Check sheet for the modelled part. Datum: model origin and axes. Units: mm. Face numbers are marked on the shaded views. Give positions to 0.01 mm unless a question says otherwise; leave off trailing zeros. Order: outer loops, then holes, each group sorted by start corner. A loop starts at its lowest first (then second) coordinate and runs counter-clockwise, first axis right, second up. Notation, with made-up numbers: (-27.75, -19.5) -> (26.25, -19.5) arc R25 cw to (26.25, 18.5) -> close; hole circle Ø9 at (-9, 50). An arc over 180 degrees is marked (long way). Answer in a Markdown table with one row per item. Add a question column.
(1) Go/stop test with flat-tipped pins: pin 1 (10 mm diameter, centred on y = 25, z = -4, fed in from +X); pin 2 (4 mm diameter, centred on y = 65, z = -6.5, fed in from -X); pin 3 (4 mm diameter, centred on x = 38, z = -4.5, fed in from -Y); pin 4 (1 mm diameter, centred on x = 30.5, z = -5.5, fed in from +Y). Record where each tip stops, or that it passes through.
(2) Thickness scan on L1, parallel to Y at x = 28.5, z = 2.5; L2, parallel to Y at x = -18.3, z = -4; L3, parallel to Z at x = 38.2, y = 62.3 (3 decimals). Record the ranges inside material, lowest first. Write a range as [from, to].
(3) Cross-section at A-A (x = 18.9). Record the cut outline in (y, z) (3 decimals), then the cut area to 3 significant figures.
(4) Cross-section at C-C (x = 27.5). Record the cut outline in (y, z) (3 decimals), then the cut area to 3 significant figures.
(5) Release check for a two-part mould opening along Y. For the marked faces 1, 2 and 3 record: released by +Y, released by -Y, zero draft, split by the parting line, or undercut.
(6) Cross-section at D-D (y = 23). Record the cut outline in (x, z), then the cut area to 3 significant figures.
(7) Cross-section at B-B (y = 39). Record the cut outline in (x, z).
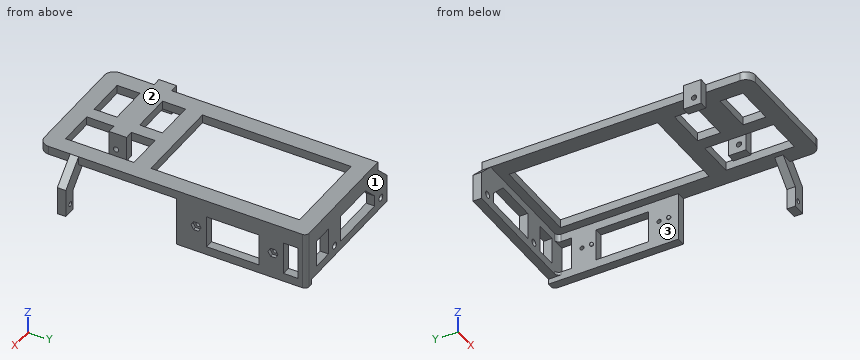
```python
from build123d import *

# Parameters (mm, degrees)
EXTRUDE_5_DEPTH      = 4
SKETCH_5_W           = 65.55
SKETCH_5_H           = 20.755
SKETCH_5_R           = 1.55
EXTRUDE_6_DEPTH      = 4
SKETCH_7_W           = 65.55
SKETCH_7_H           = 126.45
EXTRUDE_8_DEPTH      = 4
SKETCH_11_W          = 17.25
SKETCH_11_H          = 32.3
SKETCH_11_W_2        = 18.8
SKETCH_11_H_2        = 10.8
CUT_EXTRUDE_3_DEPTH  = 125.085535116
EXTRUDE_9_DEPTH      = 4
CUT_EXTRUDE_4_DEPTH  = 10
SKETCH_14_W          = 9.75
SKETCH_14_H          = 12.755
CUT_EXTRUDE_5_DEPTH  = 10
SKETCH_16_W          = 15.255
SKETCH_16_H          = 24.75
SKETCH_16_W_2        = 15.505
SKETCH_16_H_2        = 6.88
CUT_EXTRUDE_6_DEPTH  = 133.101854737
EXTRUDE_2_DEPTH      = 4
CUT_EXTRUDE_7_REACH  = 127.39
SKETCH_19_R          = 1.1
SKETCH_21_W          = 4
SKETCH_21_H          = 2.5
EXTRUDE_11_DEPTH     = 4
FILLET_2_R           = 2
FILLET_3_R           = 4.65
SKETCH_24_R          = 1
CUT_EXTRUDE_10_DEPTH = 133.101854737
SKETCH_25_R          = 0.9
EXTRUDE_12_DEPTH     = 1
FILLET_4_R           = 0.8
CUT_EXTRUDE_11_DEPTH = 1.68


with BuildPart() as part:
    # 草图4 → 凸台-拉伸5 (new body)
    with BuildSketch(Plane(origin=(37.65, 0, 0), x_dir=(0, 0, -1), z_dir=(1, 0, 0))):
        Polygon((23.255, 110.55), (19.873443934, 110.55), (11.636556066, 110.55), (0, 110.55), (0, 53.1366), (23.255, 53.1366), align=None)
    extrude(amount=EXTRUDE_5_DEPTH)

    # 草图5 → 凸台-拉伸6 (add)
    with BuildSketch(Plane(origin=(0, 110.55, 0), x_dir=(1, 0, 0), z_dir=(0, 1, 0))):
        with Locations((8.875, 10.3775)):
            Rectangle(SKETCH_5_W, SKETCH_5_H)
        with Locations(Location((-18.9, 15.755, 0), (0, 0, 180))):
            Circle(SKETCH_5_R, mode=Mode.SUBTRACT)
        with Locations(Location((18.9, 15.755, 0), (0, 0, 180))):
            Circle(SKETCH_5_R, mode=Mode.SUBTRACT)
    extrude(amount=EXTRUDE_6_DEPTH)

    # 草图7 → 凸台-拉伸8 (add)
    with BuildSketch(Plane.XY):
        with Locations((8.875, 51.325)):
            Rectangle(SKETCH_7_W, SKETCH_7_H)
    extrude(amount=EXTRUDE_8_DEPTH)

    # 草图11 → 切除-拉伸3 (cut, through all)
    with BuildSketch(Plane(origin=(0, 0, 0), x_dir=(-1, 0, 0), z_dir=(0, 0, -1))):
        with Locations((-25.025, 12.25)):
            Rectangle(SKETCH_11_W, SKETCH_11_H)
        Polygon((-33.65, 106.55), (-33.65, 36.4), (-16.4, 36.4), (8.4, 36.4), (8.4, 106.55), align=None)
        with Locations((-1, 1.5)):
            Rectangle(SKETCH_11_W_2, SKETCH_11_H_2)
        with Locations((-1, 23)):
            Rectangle(SKETCH_11_W_2, SKETCH_11_H_2)
        with BuildLine():
            ThreePointArc((16.4, -7.25), (15.038046533, -10.538046533), (11.75, -11.9))
            Line((11.75, -11.9), (23.9, -11.9))
            Line((23.9, -11.9), (23.9, 106.55))
            Line((23.9, 106.55), (16.4, 106.55))
            Line((16.4, 106.55), (16.4, -7.25))
        make_face()
    extrude(amount=-CUT_EXTRUDE_3_DEPTH, mode=Mode.SUBTRACT)

    # 草图12 → 凸台-拉伸9 (add)
    with BuildSketch(Plane(origin=(0, 2.890336251, 0), x_dir=(1, 0, 0), z_dir=(0, 1, 0))):
        Polygon((52.095757056, 19.755), (46.095757056, 19.755), (46.095757056, 9.855), (36.240757056, 0), (41.65, -4), (52.095757056, 6.445757056), align=None)
    extrude(amount=EXTRUDE_9_DEPTH)

    # 草图13 → 切除-拉伸4 (cut, symmetric)
    with BuildSketch(Plane.XZ.offset(-110.55)):
        Polygon((-23.9, -7.5), (-16.4, 0), (-16.4, 4), (-23.9, 4), align=None)
    extrude(amount=CUT_EXTRUDE_4_DEPTH, both=True, mode=Mode.SUBTRACT)

    # 草图14 → 切除-拉伸5 (cut)
    with BuildSketch(Plane.XZ.offset(-110.55)):
        with Locations((28.775, -10.3775)):
            Rectangle(SKETCH_14_W, SKETCH_14_H)
        Polygon((13.9, -16.755), (-13.9, -16.755), (-13.9, -11.642135624), (-6.257864376, -4), (13.9, -4), align=None)
    extrude(amount=-CUT_EXTRUDE_5_DEPTH, mode=Mode.SUBTRACT)

    # 草图16 → 切除-拉伸6 (cut, through all)
    with BuildSketch(Plane.ZY.offset(-37.65)):
        with Locations((-11.6275, 79.675)):
            Rectangle(SKETCH_16_W, SKETCH_16_H)
        with Locations((-11.5025, 107.11)):
            Rectangle(SKETCH_16_W_2, SKETCH_16_H_2)
    extrude(amount=-CUT_EXTRUDE_6_DEPTH, mode=Mode.SUBTRACT)

    # 草图2 → 凸台-拉伸2 (add)
    with BuildSketch(Plane.ZY.offset(16.4)):
        Polygon((-8, 12.25), (-8, 8.9), (4, 8.9), (4, 17.25), (-8, 17.25), align=None)
        with BuildLine():
            ThreePointArc((-2.75, 12.25), (-4, 11), (-5.25, 12.25))
            ThreePointArc((-5.25, 12.25), (-4, 13.5), (-2.75, 12.25))
        make_face(mode=Mode.SUBTRACT)
    extrude_2 = extrude(amount=EXTRUDE_2_DEPTH)

    # 镜向10: 凸台-拉伸2 across plane
    add(extrude_2.mirror(Plane(origin=(0, 0, 0), x_dir=(0, 0, 1), z_dir=(1, 0, 0))))

    # 草图19 → 切除-拉伸7 (cut, up to next)
    with BuildSketch(Plane.XZ.offset(-2.890336251), mode=Mode.PRIVATE) as cut_extrude_7_sk1:
        with Locations((48.495757056, -15.755)):
            Circle(SKETCH_19_R)
    cut_extrude_7_tool1 = extrude(cut_extrude_7_sk1.sketch, amount=-CUT_EXTRUDE_7_REACH, mode=Mode.PRIVATE) & part.part
    add(cut_extrude_7_tool1.solids().sort_by_distance((48.495757, 2.890336, -15.755))[0], mode=Mode.SUBTRACT)

    # 草图21 → 凸台-拉伸11 (add)
    with BuildSketch(Plane(origin=(0, 110.55, 0), x_dir=(1, 0, 0), z_dir=(0, 1, 0))):
        with Locations((39.65, 22.005)):
            Rectangle(SKETCH_21_W, SKETCH_21_H)
    extrude(amount=EXTRUDE_11_DEPTH)

    # 圆角2
    fillet_2_edges = [part.edges().sort_by_distance(p)[0] for p in [
        (37.65, 110.55, -20.005),
        (41.65, 114.55, -9.6275),
        (37.65, 110.55, -1.875),
    ]]
    fillet(fillet_2_edges, radius=FILLET_2_R)

    # 圆角3
    fillet_3_edges = [part.edges().sort_by_distance(p)[0] for p in [
        (41.65, -11.9, 2),
    ]]
    fillet(fillet_3_edges, radius=FILLET_3_R)

    # 草图24 → 切除-拉伸10 (cut, through all)
    with BuildSketch(Plane.ZY.offset(-37.65)):
        with Locations(Location((-10.755, 62.3, 0), (0, 0, 270))):
            Circle(SKETCH_24_R)
        with Locations(Location((-10.755, 98.67, 0), (0, 0, 270))):
            Circle(SKETCH_24_R)
    extrude(amount=-CUT_EXTRUDE_10_DEPTH, mode=Mode.SUBTRACT)

    # 草图25 → 凸台-拉伸12 (add)
    with BuildSketch(Plane.ZY.offset(-37.65)):
        with Locations(Location((-10.755, 57.65, 0), (0, 0, 90))):
            Circle(SKETCH_25_R)
        with Locations(Location((-10.755, 94.05, 0), (0, 0, 90))):
            Circle(SKETCH_25_R)
    extrude(amount=EXTRUDE_12_DEPTH)

    # 圆角4
    fillet_4_edges = [part.edges().sort_by_distance(p)[0] for p in [
        (36.65, 93.15, -10.755),
        (36.65, 56.75, -10.755),
    ]]
    fillet(fillet_4_edges, radius=FILLET_4_R)

    # 草图27 → 切除-拉伸11 (cut)
    with BuildSketch(Plane(origin=(41.65, 0, 0), x_dir=(0, 0, -1), z_dir=(1, 0, 0))):
        Polygon((10.755, 96.302863896), (12.805, 97.486431948), (12.805, 99.853568052), (10.755, 101.037136104), (8.705, 99.853568052), (8.705, 97.486431948), align=None)
        Polygon((10.755, 59.932863896), (12.805, 61.116431948), (12.805, 63.483568052), (10.755, 64.667136104), (8.705, 63.483568052), (8.705, 61.116431948), align=None)
    extrude(amount=-CUT_EXTRUDE_11_DEPTH, mode=Mode.SUBTRACT)


solid = part.part
```
Answer below:
| question | item | result |
|---|---|---|
| 1 | pin 1 | stops at x = 41.65 |
| 1 | pin 2 | stops at x = 37.65 |
| 1 | pin 3 | stops at y = 2.89 |
| 1 | pin 4 | passes through |
| 2 | L1 | y = [-11.9, -3.9], [28.4, 36.4], [106.55, 114.55] |
| 2 | L2 | y = [8.9, 11], [13.5, 17.25], [110.55, 114.55] |
| 2 | L3 | z = [-23.255, -11.755], [-9.755, 4] |
| 3 | outline | (-11.9, 0) -> (-3.9, 0) -> (-3.9, 4) -> (-11.9, 4) -> close; (8.9, -8) -> (17.25, -8) -> (17.25, 4) -> (8.9, 4) -> close; (28.4, 0) -> (36.4, 0) -> (36.4, 4) -> (28.4, 4) -> close; (106.55, 0) -> (110.55, 0) -> (110.55, -14.205) -> (114.55, -14.205) -> (114.55, 4) -> (106.55, 4) -> close; (110.55, -20.755) -> (114.55, -20.755) -> (114.55, -17.305) -> (110.55, -17.305) -> close; hole circle Ø2.5 at (12.25, -4) |
| 3 | area | 262 mm² |
| 4 | outline | (-11.9, 0) -> (-3.9, 0) -> (-3.9, 4) -> (-11.9, 4) -> close; (28.4, 0) -> (36.4, 0) -> (36.4, 4) -> (28.4, 4) -> close; (106.55, 0) -> (110.55, 0) -> (110.55, -4) -> (114.55, -4) -> (114.55, 4) -> (106.55, 4) -> close; (110.55, -20.755) -> (114.55, -20.755) -> (114.55, -16.755) -> (110.55, -16.755) -> close |
| 4 | area | 128 mm² |
| 5 | face 1 | released by +Y |
| 5 | face 2 | zero draft |
| 5 | face 3 | undercut |
| 6 | outline | (-16.4, 0) -> (-8.4, 0) -> (-8.4, 4) -> (-16.4, 4) -> close; (10.4, 0) -> (16.4, 0) -> (16.4, 4) -> (10.4, 4) -> close; (33.65, 0) -> (41.65, 0) -> (41.65, 4) -> (33.65, 4) -> close |
| 6 | area | 88.0 mm² |
| 7 | outline | (-16.4, 0) -> (-8.4, 0) -> (-8.4, 4) -> (-16.4, 4) -> close; (33.65, 0) -> (41.65, 0) -> (41.65, 4) -> (33.65, 4) -> close |
